Verification items for this drawing (mm, ordinates from the low corner). A direction names the side the tool comes from. Coordinates: 2 decimals unless noted, no trailing zeros. Order: outer loops, then holes, each group sorted by start corner. A loop starts at its lowest first (then second) coordinate and runs counter-clockwise, first axis right, second up. Notation, with made-up numbers: (41.25, 73) -> (89.25, 73) arc R17 cw to (89.25, 94) -> close; hole circle Ø7 at (41.5, 19). An arc over 180 degrees is marked (long way). Write item = value, one per line. Start each with the question number.
1. Cross-section at B-B on y = 5. Record the cut outline in (x, z).
2. Cross-section at D-D on z = 5. Record the cut outline in (x, y), plus the area to 3 significant figures.
3. Thickness scan on line 1 along Z through (x, y) = (25.5, 5); line 2 along X through (y, z) = (5, 4.5); line 3 along X through (y, z) = (6.25, 4.5). Record the ranges inside material, lowest first. Write a range as from..to.
4. Release check for a two-part mould opening along Z. For the marked faces 1, 2 and 3 record: +Z half, -Z half, draft (parallel to the pull), parting line (faces both ways), or undercut.
5. Set-up check for the marked faces 4 and 5: record each of +Z, -Z, +X, -X, +Y, -Y from which the full face is reachable in a straight line by a thin tool's end or side.
6. Go/stop test with flat-tipped pins: P1, Ø0.6, axis at y = 7, z = 6, coming from the -X side; P2, Ø0.6, axis at y = 7, z = 1, coming from the +X side; P3, Ø6, axis at x = 13, y = 7.5, coming from the +Z side; P4, Ø4, axis at x = 19, y = 6, coming from the -Z side. Record where each tip stops, or that it passes through.
7. Cross-section at A-A on x = 25.5. Record the cut outline in (y, z).
8. Cross-section at C-C on z = 3.5. Record the cut outline in (x, y).
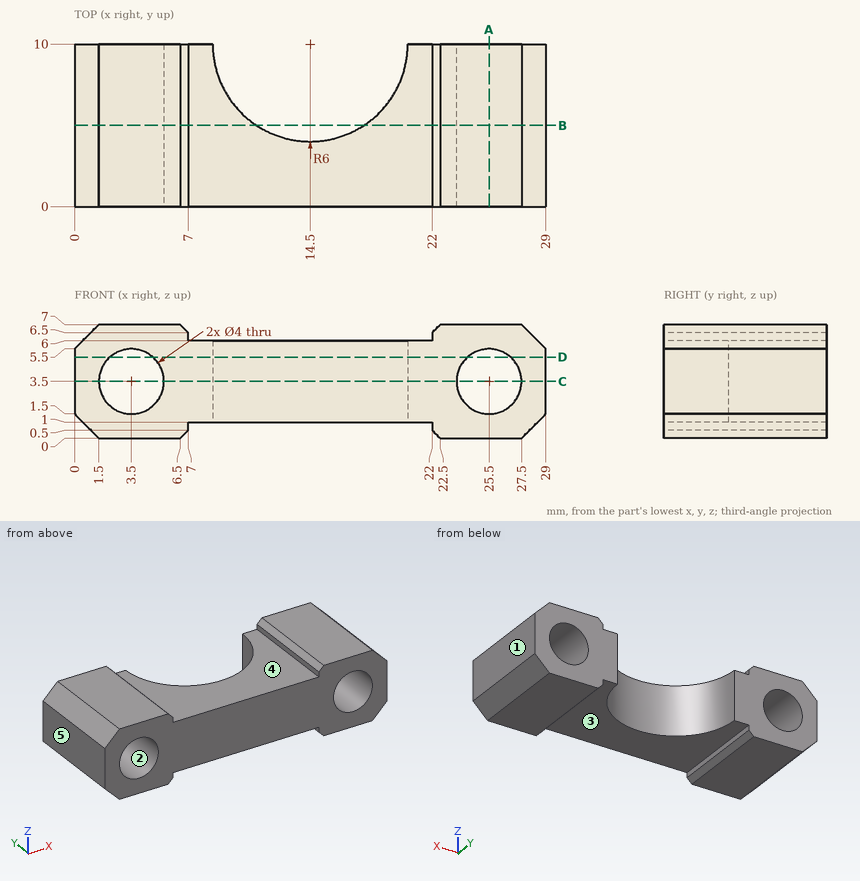
Worked out:
q1.outline = (0, 1.5) -> (1.5, 0) -> (6.5, 0) -> (7, 0.5) -> (7, 1) -> (11.18, 1) -> (11.18, 6) -> (7, 6) -> (7, 6.5) -> (6.5, 7) -> (1.5, 7) -> (0, 5.5) -> close; (17.82, 1) -> (22, 1) -> (22, 0.5) -> (22.5, 0) -> (27.5, 0) -> (29, 1.5) -> (29, 5.5) -> (27.5, 7) -> (22.5, 7) -> (22, 6.5) -> (22, 6) -> (17.82, 6) -> close; hole circle Ø4 at (3.5, 3.5); hole circle Ø4 at (25.5, 3.5)
q2.outline = (0, 0) -> (2.18, 0) -> (2.18, 10) -> (0, 10) -> close; (4.82, 0) -> (24.18, 0) -> (24.18, 10) -> (20.5, 10) arc R6 cw to (8.5, 10) -> (4.82, 10) -> close; (26.82, 0) -> (29, 0) -> (29, 10) -> (26.82, 10) -> close
q2.area = 181 mm²
q3.line_1 = 0..1.5, 5.5..7
q3.line_2 = 0..1.77, 5.23..11.18, 17.82..23.77, 27.23..29
q3.line_3 = 0..1.77, 5.23..9.82, 19.18..23.77, 27.23..29
q4.face_1 = draft
q4.face_2 = undercut
q4.face_3 = -Z half
q5.face_4 = +Z, +Y, -Y
q5.face_5 = +Z, -Z, -X, +Y, -Y
q6.P1 = 0.2
q6.P2 = 28.8
q6.P3 = through
q6.P4 = 1
q7.outline = (0, 0) -> (10, 0) -> (10, 1.5) -> (0, 1.5) -> close; (0, 5.5) -> (10, 5.5) -> (10, 7) -> (0, 7) -> close
q8.outline = (0, 0) -> (1.5, 0) -> (1.5, 10) -> (0, 10) -> close; (5.5, 0) -> (23.5, 0) -> (23.5, 10) -> (20.5, 10) arc R6 cw to (8.5, 10) -> (5.5, 10) -> close; (27.5, 0) -> (29, 0) -> (29, 10) -> (27.5, 10) -> close
